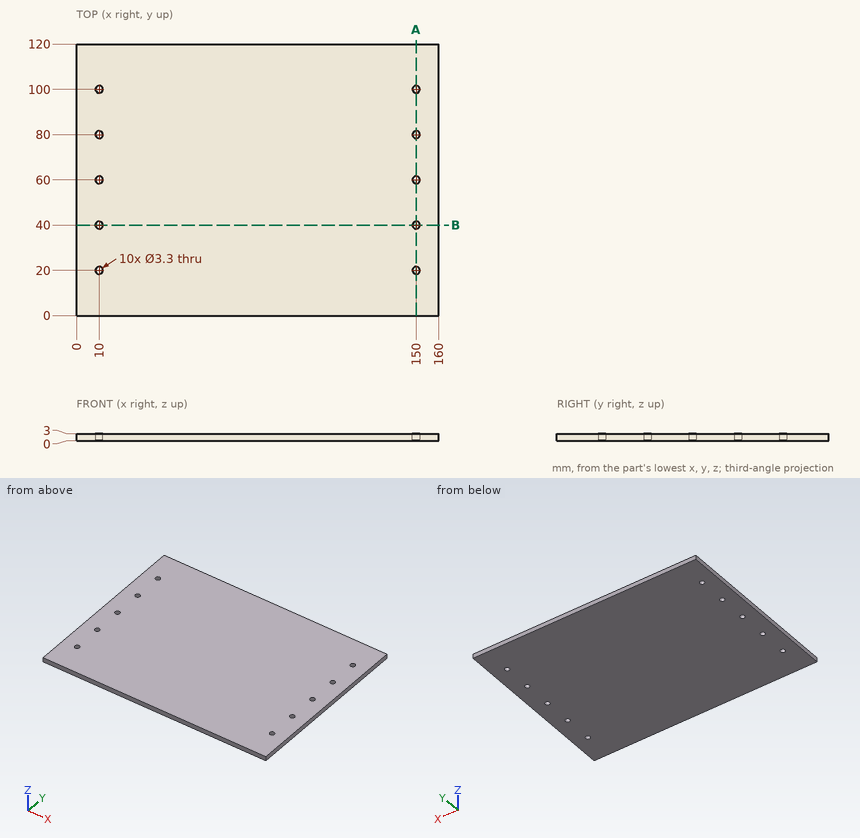
Could you check a few things on this drawing? It's one solid part, dimensions in mm from its lowest x, y, z. Give positions to 0.01 mm unless a question says otherwise; leave off trailing zeros. Write each loop counter-clockwise with the first axis right and the second up, starting at its lowest first coordinate (ties: lowest second). Pieces come first, ordered by that corner, then holes. Notation, with made-up numbers: M 58.25,-34.5 L 73.25,-34.5 A14 cw 73.25,-13.5 Z; hole C 25,46 d1. An arc over 180 degrees is marked long. Put each result on its own line as item: value. Start each with the question number.
Item 1: Will these pins go through, and if not, where does the flat tip stop? pin 1 (4.5 mm diameter, centred on x = 10, y = 80, fed in from -Z); pin 2 (2 mm diameter, centred on x = 10, y = 20, fed in from +Z).
Item 2: If we section it at B-B, the plane y = 40: Write out the boundary of the cut face in (x, z).
Item 3: If we section it at A-A, the plane x = 150: Write out the boundary of the cut face in (y, z).
Item 4: I need wall thicknesses on L1, parallel to Y at x = 150, z = 0.75; L2, parallel to X at y = 80, z = 1.75. Which ranges of each line are inside material? Lowest first, please. Write a range as from..to.
Values:
1. pin 1: z = 0
1. pin 2: through
2. outline: M 0,0 L 8.35,0 L 8.35,3 L 0,3 Z; M 11.65,0 L 148.35,0 L 148.35,3 L 11.65,3 Z; M 151.65,0 L 160,0 L 160,3 L 151.65,3 Z
3. outline: M 0,0 L 18.35,0 L 18.35,3 L 0,3 Z; M 21.65,0 L 38.35,0 L 38.35,3 L 21.65,3 Z; M 41.65,0 L 58.35,0 L 58.35,3 L 41.65,3 Z; M 61.65,0 L 78.35,0 L 78.35,3 L 61.65,3 Z; M 81.65,0 L 98.35,0 L 98.35,3 L 81.65,3 Z; M 101.65,0 L 120,0 L 120,3 L 101.65,3 Z
4. L1: 0..18.35, 21.65..38.35, 41.65..58.35, 61.65..78.35, 81.65..98.35, 101.65..120
4. L2: 0..8.35, 11.65..148.35, 151.65..160
